Geometry check sheet. Reference: the model listing, model coordinates, mm. A direction names the side the tool comes from. Give positions to 0.01 mm unless a question says otherwise; leave off trailing zeros. Order: outer loops, then holes, each group sorted by start corner. A loop starts at its lowest first (then second) coordinate and runs counter-clockwise, first axis right, second up. Notation, with made-up numbers: (12.5, 70) - (38.5, 70) arc R19 cw to (38.5, 106) - close; hole circle Ø9 at (53, 62.5). An arc over 180 degrees is marked (long way). Put each result on its own line as item: value. Start each with the question number.
```python
from build123d import *

# Parameters (mm, degrees)
SKETCH1_W           = 27.15
SKETCH1_H           = 11.75
BOSS_EXTRUDE1_DEPTH = 4
SKETCH2_W           = 21.9
SKETCH2_H           = 11.75
BOSS_EXTRUDE2_DEPTH = 1.25
BOSS_EXTRUDE2_TAPER = 5


with BuildPart() as part:
    # Sketch1 → Boss-Extrude1 (new body)
    with BuildSketch(Plane.XY):
        Rectangle(SKETCH1_W, SKETCH1_H)
    extrude(amount=BOSS_EXTRUDE1_DEPTH)

    # Sketch2 → Boss-Extrude2 (add)
    with BuildSketch(Plane.XY.offset(4)):
        with Locations((-2.625, 0)):
            Rectangle(SKETCH2_W, SKETCH2_H)
    extrude(amount=BOSS_EXTRUDE2_DEPTH, taper=BOSS_EXTRUDE2_TAPER)


solid = part.part
```
Item 1: Set-up check for faces 1 (the face through (11, 0, 4)), 2 (the face through (-13.52, -0.08, 4.62)): record each of +Z, -Z, +X, -X, +Y, -Y from which the full face is reachable in a straight line by a thin tool's end or side.
Item 2: Release check for a two-part mould opening along Y. For faces 3 (the face through (0, -5.875, 2)), 4 (the face through (-2.78, 5.82, 4.62)), 5 (the face through (-3, 0, 5.25)) record: +Y half, -Y half, draft (parallel to the pull), parting line (faces both ways), or undercut.
Item 3: Cross-section at A-A (y = -4). Enter the section's corners in (x, z) (3 decimals).
Item 4: Cross-section at C-C (z = 4.75). Enter the section's corners in (x, y).
Item 5: Gauge pin test, flat end, axial feed: pin 1 Ø4 at (x, y) = (11, 0) entering from +Z. Record the tip position at first contact, or that the pin passes through.
Item 6: Cross-section at B-B (x = 9.5). Enter the section's corners in (y, z) (3 decimals), and give its area (3 significant figures).
Item 7: Thickness scan on line 1 along Z through (x, y) = (9.25, 3.25); line 2 along Y through (x, z) = (-2.5, 4.1); line 3 along X through (y, z) = (-4, 4.15). Record the ranges inside material, lowest first.
Recorded:
1. face 1: +Z, +X, +Y, -Y
1. face 2: +Z, -X, +Y, -Y
2. face 3: -Y half
2. face 4: +Y half
2. face 5: draft
3. outline: (-13.575, 0) - (13.575, 0) - (13.575, 4) - (8.325, 4) - (8.216, 5.25) - (-13.466, 5.25) - (-13.575, 4) - close
4. outline: (-13.51, -5.81) - (8.26, -5.81) - (8.26, 5.81) - (-13.51, 5.81) - close
5. pin 1: stops at z = 4
6. outline: (-5.875, 0) - (5.875, 0) - (5.875, 4) - (-5.875, 4) - close
6. area: 47.0 mm^2
7. line 1: z = 0 to 4
7. line 2: y = -5.87 to 5.87
7. line 3: x = -13.56 to 8.31
